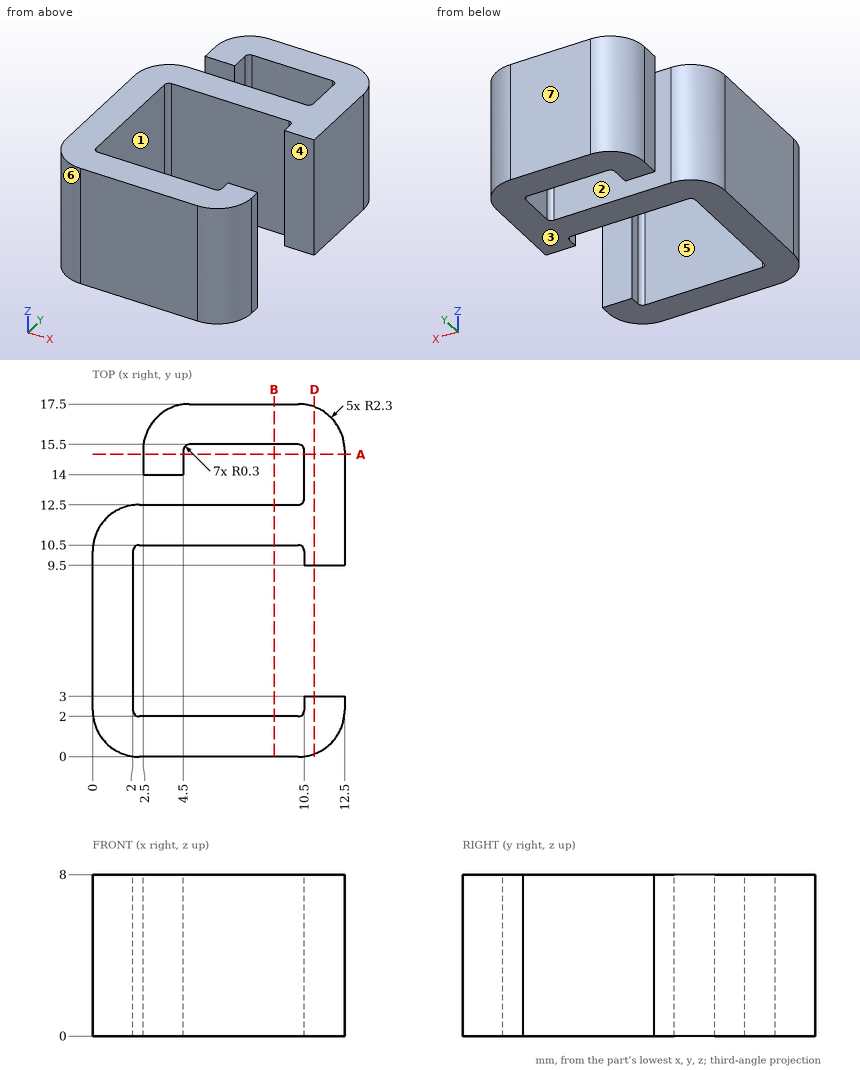
Geometry check sheet. Reference: drawing and pictorial views, mm from the part's lowest x, y, z. A direction names the side the tool comes from. Give positions to 0.01 mm unless a question says otherwise; leave off trailing zeros. Order: outer loops, then holes, each group sorted by start corner. A loop starts at its lowest first (then second) coordinate and runs counter-clockwise, first axis right, second up. Notation, with made-up numbers: (27.5, -24) - (75.5, -24) arc R35 ccw to (75.5, 10) - close; hole circle Ø5 at (-12, 38). An arc over 180 degrees is marked (long way). Answer as CSV lines item,"result". Start each with the question number.
Item 1: Gauge pin test, flat ends, axial feed: pin 1 (1.6 mm diameter, centred on x = 11.5, z = 5, fed in from -Y) (3 decimals); pin 2 (4 mm diameter, centred on y = 6, z = 6, fed in from +X); pin 3 (1 mm diameter, centred on x = 11.5, z = 3, fed in from +Y). Record the tip position at first contact, or that the pin passes through.
Item 2: Section check D-D, the plane x = 11. Record the boundary of the cut face in (y, z), plus the area to 3 significant figures.
Item 3: Access from +Z, -Z, +X, -X, +Y, -Y to the whole of each face (thin tool, end or side, straight path). Record for the marked faces 1, 2, 3 and 4.
Item 4: Section check B-B, the plane x = 9. Record the boundary of the cut face in (y, z).
Item 5: Mould release check, pull along X, two halves, no side actions. Record for the marked faces 5, 6 and 7: released by +X, released by -X, zero draft, split by the parting line, or undercut.
Item 6: Section check A-A, the plane y = 15. Record the boundary of the cut face in (x, z).
Item 7: Material ranges on L1, parallel to Y at x = 8.75, z = 1.5; L2, parallel to X at y = 14.5, z = 3.25; L3, parallel to Y at x = 3.75, z = 7, recorded low to high.
Filled in:
1,pin 1,"y = 0.055"
1,pin 2,"x = 2"
1,pin 3,"y = 17.36"
2,outline,"(0.14, 0) - (3, 0) - (3, 8) - (0.14, 8) - close; (9.5, 0) - (17.36, 0) - (17.36, 8) - (9.5, 8) - close"
2,area,"85.7 mm^2"
3,face 1,"+Z, -Z"
3,face 2,"+Z, -Z, -X"
3,face 3,"-Z, +X, -X, +Y, -Y"
3,face 4,"+Z, -Z, +X"
4,outline,"(0, 0) - (2, 0) - (2, 8) - (0, 8) - close; (10.5, 0) - (12.5, 0) - (12.5, 8) - (10.5, 8) - close; (15.5, 0) - (17.5, 0) - (17.5, 8) - (15.5, 8) - close"
5,face 5,"undercut"
5,face 6,"released by -X"
5,face 7,"zero draft"
6,outline,"(2.5, 0) - (4.5, 0) - (4.5, 8) - (2.5, 8) - close; (10.5, 0) - (12.5, 0) - (12.5, 8) - (10.5, 8) - close"
7,L1,"0 to 2, 10.5 to 12.5, 15.5 to 17.5"
7,L2,"2.5 to 4.5, 10.5 to 12.5"
7,L3,"0 to 2, 10.5 to 12.5, 14 to 17.25"
